from build123d import *

# Parameters (mm, degrees)
SKETCH_1_R               = 3.24
EXTRUDE_1_DEPTH          = 2
SKETCH_2_R               = 5.25
SKETCH_2_R_2             = 3.25
EXTRUDE_2_DEPTH          = 90
CUT_EXTRUDE_1_DEPTH      = 54.547292182
CUT_EXTRUDE_1_DEPTH_BACK = 54.547292182


with BuildPart() as part:
    # Эскиз1 → Бобышка-Вытянуть1 (new body)
    with BuildSketch(Plane(origin=(0, 0, 0), x_dir=(1, 0, 0), z_dir=(0, 1, 0))):
        with BuildLine():
            Line((-25, 22.5), (25, 22.5))
            ThreePointArc((25, 22.5), (39.142135624, 16.642135624), (45, 2.5))
            Line((45, 2.5), (45, -22.5))
            Line((45, -22.5), (-45, -22.5))
            Line((-45, -22.5), (-45, 2.5))
            ThreePointArc((-45, 2.5), (-39.142135624, 16.642135624), (-25, 22.5))
        make_face()
        with Locations(Location((-28.24, -7.5, 0), (0, 0, 270))):
            Circle(SKETCH_1_R, mode=Mode.SUBTRACT)
        with Locations(Location((-15, 12.5, 0), (0, 0, 270))):
            Circle(SKETCH_1_R, mode=Mode.SUBTRACT)
        with Locations(Location((15, 12.5, 0), (0, 0, 90))):
            Circle(SKETCH_1_R, mode=Mode.SUBTRACT)
        with Locations(Location((28.24, -7.5, 0), (0, 0, 90))):
            Circle(SKETCH_1_R, mode=Mode.SUBTRACT)
    extrude(amount=EXTRUDE_1_DEPTH)

    # Эскиз2 → Бобышка-Вытянуть2 (add)
    with BuildSketch(Plane(origin=(45, 0, 0), x_dir=(0, 0, -1), z_dir=(1, 0, 0))):
        with Locations((-22.5, 5.25)):
            Circle(SKETCH_2_R)
        with Locations((-22.5, 5.25)):
            Circle(SKETCH_2_R_2, mode=Mode.SUBTRACT)
    extrude(amount=-EXTRUDE_2_DEPTH)

    # Эскиз3 → Вырез-Вытянуть1 (cut, two sides: drawn at the far end of the back side and taken through both)
    with BuildSketch(Plane(origin=(0, 2, 0), x_dir=(1, 0, 0), z_dir=(0, 1, 0)).offset(-CUT_EXTRUDE_1_DEPTH_BACK)):
        with BuildLine():
            Line((-21.495, -40.75), (21.495, -40.75))
            Line((21.495, -40.75), (21.495, -17.25))
            ThreePointArc((21.495, -17.25), (20.762766953, -15.482233047), (18.995, -14.75))
            Line((18.995, -14.75), (-18.995, -14.75))
            ThreePointArc((-18.995, -14.75), (-20.762766953, -15.482233047), (-21.495, -17.25))
            Line((-21.495, -17.25), (-21.495, -40.75))
        make_face()
    extrude(amount=CUT_EXTRUDE_1_DEPTH + CUT_EXTRUDE_1_DEPTH_BACK, mode=Mode.SUBTRACT)


solid = part.part
Source: CAD feature listing. Evaluate the final solid. Frame: model axes, mm. A direction names the side the tool comes from. Round coordinates to 2 decimals unless told otherwise and drop trailing zeros. Write each loop counter-clockwise with the first axis right and the second up, starting at its lowest first coordinate (ties: lowest second). Pieces come first, ordered by that corner, then holes. Notation, with made-up numbers: (47.5, 49) - (51.5, 49) arc R30 ccw to (51.5, 79) - close; hole circle Ø10 at (70, -8). An arc over 180 degrees is marked (long way). Use CSV: the item, a comma, the result in double quotes. Start each with the question number.
(1) First-contact query: pin 1 Ø6 at (x, z) = (-1.5, -16) entering from +Y; pin 2 Ø1.6 at (x, y) = (-4, 1) entering from +Z. Flat tips, straight axial feed; report the tip coordinate or a pass-through.
(2) Material intervals for probe 1 along X at (y, z) = (1.5, 18) (3 decimals); probe 2 along X at (y, z) = (0.45, 7.5); probe 3 along X at (y, z) = (1.3, -12.5), sorted ascending. Write a range as [from, to].
(3) Cut plane C-C, the plane z = -12.5. Return loops of the section in (x, y).
(4) Cut plane B-B, the plane y = 5.25. Return loops of the section in (x, z) (3 decimals), and give its area (3 significant figures).
(5) Set-up query: faces 1 (the face through (21.495, 5, 19)), 2 (the face through (-45, 1.8, 17.2)). Return all of +Z, -Z, +X, -X, +Y, -Y with unobstructed straight access to the full face (end or side cutting, diameter ignored); none if empty.
(6) Cut plane D-D, the plane x = -28.24. Return loops of the section in (y, z).
(7) Cut plane A-A, the plane x = -15. Return loops of the section in (y, z), and give its area (3 significant figures).
(8) Mould query, pull axis Z, two halves, no side actions, for faces 3 (the face through (0, 1, -22.5)), 4 (the face through (1, 0, 0)), 5 (the face through (-31.403, 0.986, 6.798)). Classes: pulls with the +Z half, pulls with the -Z half, needs draft (parallel to the pull), parting line crosses it, or undercut.
Geometry says:
1,pin 1,"y = 2"
1,pin 2,"z = 14.75"
2,probe 1,"[-45, -21.495], [21.495, 45]"
2,probe 2,"[-45, -31.48], [-25, 25], [31.48, 45]"
2,probe 3,"[-42.32, -18.24], [-11.76, 11.76], [18.24, 42.32]"
3,outline,"(-42.32, 0) - (-18.24, 0) - (-18.24, 2) - (-42.32, 2) - close; (-11.76, 0) - (11.76, 0) - (11.76, 2) - (-11.76, 2) - close; (18.24, 0) - (42.32, 0) - (42.32, 2) - (18.24, 2) - close"
4,outline,"(-45, 17.25) - (-21.495, 17.25) - (-21.495, 19.25) - (-45, 19.25) - close; (-45, 25.75) - (-21.495, 25.75) - (-21.495, 27.75) - (-45, 27.75) - close; (21.495, 17.25) - (45, 17.25) - (45, 19.25) - (21.495, 19.25) - close; (21.495, 25.75) - (45, 25.75) - (45, 27.75) - (21.495, 27.75) - close"
4,area,"188 mm²"
5,face 1,"+Z, +Y, -Y"
5,face 2,"+Z, -Z, -X, +Y, -Y"
6,outline,"(0, -22.24) - (2, -22.24) - (2, 4.26) - (0, 4.26) - close; (0, 10.74) - (2, 10.74) - (2, 18.38) arc R5.25 ccw (long way) to (0, 22.5) - close; hole circle Ø6.5 at (5.25, 22.5)"
7,outline,"(0, -22.5) - (2, -22.5) - (2, -15.74) - (0, -15.74) - close; (0, -9.26) - (2, -9.26) - (2, 14.75) - (0, 14.75) - close"
7,area,"61.5 mm²"
8,face 3,"pulls with the -Z half"
8,face 4,"needs draft"
8,face 5,"undercut"
